Could you check a few things on this drawing? It's one solid part, dimensions in mm from its lowest x, y, z. A direction names the side the tool comes from. Round coordinates to 2 decimals unless told otherwise and drop trailing zeros. Write each loop counter-clockwise with the first axis right and the second up, starting at its lowest first coordinate (ties: lowest second). Pieces come first, ordered by that corner, then holes. Notation, with made-up numbers: M 56.5,55.25 L 96.5,55.25 A17 ccw 96.5,72.25 Z; hole C 1.5,-25.75 d7. An arc over 180 degrees is marked long. One line per item, written item: value. Start each with the question number.
(1) Thinking about a two-plate mould opening in X: for the marked faces 1, 2 and 3, which applies, released by +X, released by -X, zero draft, split by the parting line, or undercut?
(2) I want a section at C-C on y = 18.75. Please give me the cut outline in (x, z), and give its area (3 significant figures).
(3) If I drill on L1, parallel to X at y = 17.25, z = 13; L2, parallel to Y at x = 33.5, z = 19.5 (1 decimal); L3, parallel to Z at x = 35, y = 17.5, over which ranges is the centre line in solid material (lowest first)?
(4) I want a section at B-B on x = 17.5. Please give me the cut outline in (y, z) (1 decimal).
(5) Which directions (+Z, -Z, +X, -X, +Y, -Y) give clear straight access to the entire face, cutting with the end or side of a thin tool? Please do the marked faces 4 and 5.
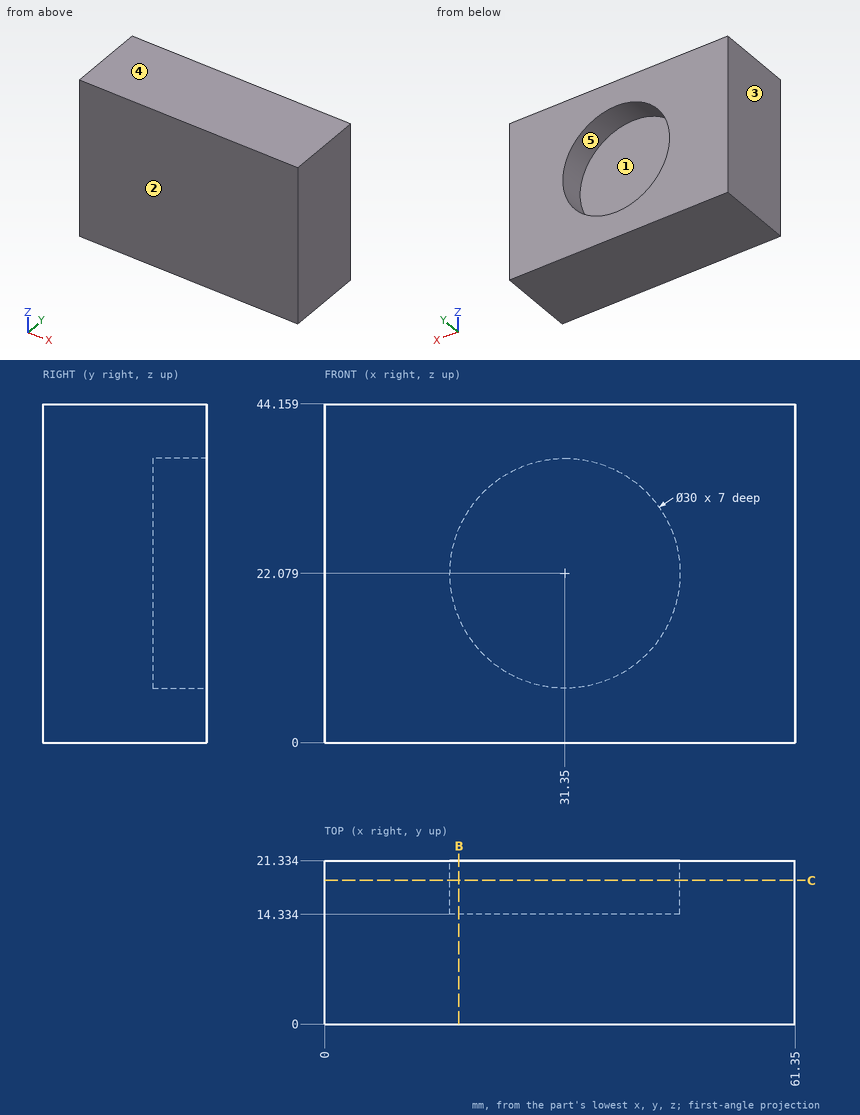
Found:
1. face 1: undercut
1. face 2: zero draft
1. face 3: released by -X
2. outline: M 0,0 L 61.35,0 L 61.35,44.16 L 0,44.16 Z; hole C 31.35,22.08 d30
2. area: 2,000 mm²
3. L1: x = 0 to 19.41, 43.29 to 61.35
3. L2: y = 0 to 14.3
3. L3: z = 0 to 7.53, 36.63 to 44.16
4. outline: M 0,0 L 21.3,0 L 21.3,16.3 L 14.3,16.3 L 14.3,27.8 L 21.3,27.8 L 21.3,44.2 L 0,44.2 Z
5. face 4: +Z, +X, -X, +Y, -Y
5. face 5: +Y
